For this review, take the finished solid that the model builds, in its own axes (mm). A direction names the side the tool comes from. Round coordinates to 2 decimals unless told otherwise and drop trailing zeros. Loops run counter-clockwise (first coordinate to the right, second up) from the corner with the lowest first, then second, coordinate; pieces in that order, holes last. Notation, with made-up numbers: M -17,66.5 L 3,66.5 A22 cw 3,75.5 Z; hole C 31,-6 d3. An arc over 180 degrees is marked long. One line per question, with ' | ' between items. Start each with the question number.
1) For probe 1 along X at (y, z) = (-49.5, 1) (3 decimals), list the stretches that pass through material, from the lowest coordinate up. Write a range as from..to.
2) We need section B-B (z = 4.25). Give the boundary of the cut face in (x, y) (1 decimal), and give its area (3 significant figures).
3) Mouldability with a two-part tool opening along X and no side actions: class faces 1 (the face through (117.475, -2, 3)), 2 (the face through (-2, 2, 0)), 3 (the face through (51, 63.5, 3)) as pulls with the +X half, pulls with the -X half, needs draft (parallel to the pull), parting line crosses it, or undercut.
4) We need section A-A (y = -46). Give the boundary of the cut face in (x, z) (3 decimals), and give its area (3 significant figures).
5) For faces 4 (the face through (-117.475, -2, 3)), 5 (the face through (-38.1, 51, 3)), list the 3-axis set-ups (+Z, -Z, +X, -X, +Y, -Y) from which the entire face can be reached by the end or side of a thin tool; tool diameter is ignored.
```python
from build123d import *

# Parameters (mm, degrees)
F0_W     = 234.95
F0_H     = 234.95
F1_DEPTH = 6.35
F2_W     = 25.4
F2_H     = 25.4
F3_DEPTH = 25.4


with BuildPart() as f1:
    # F0 (on Top) → F1 (new body)
    with BuildSketch(Plane.XY):
        Rectangle(F0_W, F0_H)
    extrude(amount=F1_DEPTH)

    # F2 (on face) → F3 (cut)
    with BuildSketch(Plane.XY.offset(6.35)):
        with Locations((-50.8, 50.8)):
            Rectangle(F2_W, F2_H)
        with Locations((50.8, 50.8)):
            Rectangle(F2_W, F2_H)
        with Locations((50.8, -50.8)):
            Rectangle(F2_W, F2_H)
        with Locations((-50.8, -50.8)):
            Rectangle(F2_W, F2_H)
        with BuildLine():
            ThreePointArc((1.5875, 0), (1.1225320151, 1.1225320151), (0, 1.5875))
            Line((0, 1.5875), (0, 0))
            Line((0, 0), (1.5875, 0))
        make_face()
        with BuildLine():
            Line((0, -1.5875), (0, 0))
            Line((0, 0), (-1.5875, 0))
            ThreePointArc((-1.5875, 0), (-1.1225320151, -1.1225320151), (0, -1.5875))
        make_face()
        with BuildLine():
            ThreePointArc((0, -1.5875), (1.1225320151, -1.1225320151), (1.5875, 0))
            Line((1.5875, 0), (0, 0))
            Line((0, 0), (0, -1.5875))
        make_face()
    extrude(amount=-F3_DEPTH, mode=Mode.SUBTRACT)


solid = f1.part
```
Answers below:
1) probe 1: -117.475..-63.5, -38.1..38.1, 63.5..117.475
2) outline: M -117.5,-117.5 L 117.5,-117.5 L 117.5,117.5 L -117.5,117.5 Z; hole M -63.5,-63.5 L -38.1,-63.5 L -38.1,-38.1 L -63.5,-38.1 Z; hole M -63.5,38.1 L -38.1,38.1 L -38.1,63.5 L -63.5,63.5 Z; hole M -1.6,0 A1.6 ccw long 0,1.6 L 0,0 Z; hole M 38.1,-63.5 L 63.5,-63.5 L 63.5,-38.1 L 38.1,-38.1 Z; hole M 38.1,38.1 L 63.5,38.1 L 63.5,63.5 L 38.1,63.5 Z | area: 52,600 mm^2
3) face 1: pulls with the +X half | face 2: needs draft | face 3: undercut
4) outline: M -117.475,0 L -63.5,0 L -63.5,6.35 L -117.475,6.35 Z; M -38.1,0 L 38.1,0 L 38.1,6.35 L -38.1,6.35 Z; M 63.5,0 L 117.475,0 L 117.475,6.35 L 63.5,6.35 Z | area: 1,170 mm^2
5) face 4: +Z, -Z, -X, +Y, -Y | face 5: +Z, -Z
